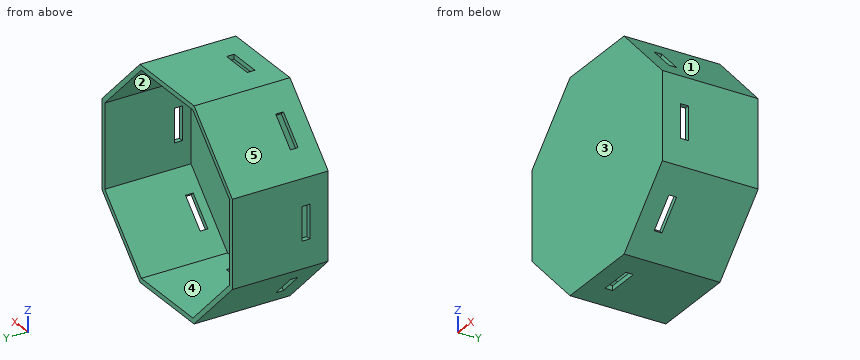
Autodesk Inventor part; units mm, degrees
ref_plane "YZ Plane" through (0, 0, 0) normal (1, 0, 0) x (0, 1, 0)
ref_plane "XZ Plane" through (0, 0, 0) normal (0, 1, 0) x (-1, 0, 0)
ref_plane "XY Plane" through (0, 0, 0) normal (0, 0, 1) x (1, 0, 0)
sketch "Skizze4" plane through (0, 0, 0) normal (0, 1, 0) x (-1, 0, 0)
  line L0 (77, 0) -> (-77, 0) construction
  line L1 (0, -77) -> (0, 77) construction
  line L2 (27, 37.5) -> (-27, 37.5) construction
  line L3 (-27, 37.5) -> (-27, -37.5) construction
  line L4 (-27, -37.5) -> (27, -37.5) construction
  line L5 (27, -37.5) -> (27, 37.5) construction
  line L6 (55, -22.7817) -> (22.7817, -55)
  line L7 (22.7817, -55) -> (-22.7817, -55)
  line L8 (-22.7817, -55) -> (-55, -22.7817)
  line L9 (-55, -22.7817) -> (-55, 22.7817)
  line L10 (-55, 22.7817) -> (-22.7817, 55)
  line L11 (-22.7817, 55) -> (22.7817, 55)
  line L12 (22.7817, 55) -> (55, 22.7817)
  line L13 (55, 22.7817) -> (55, -22.7817)
  line L14 (52.5, -21.7462) -> (21.7462, -52.5)
  line L15 (21.7462, -52.5) -> (-21.7462, -52.5)
  line L16 (-21.7462, -52.5) -> (-52.5, -21.7462)
  line L17 (-52.5, -21.7462) -> (-52.5, 21.7462)
  line L18 (-52.5, 21.7462) -> (-21.7462, 52.5)
  line L19 (-21.7462, 52.5) -> (21.7462, 52.5)
  line L20 (21.7462, 52.5) -> (52.5, 21.7462)
  line L21 (52.5, 21.7462) -> (52.5, -21.7462)
  point P0 (0, 0)
  point P1 (0, 0)
  dimension "d4" = 75
  dimension "d5" = 54
  dimension "d7" = 2.5
  dimension "d22" = 110
extrude "Extrusion2" add sketch "Skizze4" along normal blind 45
sketch "Skizze5" plane through (0, 0, 0) normal (0, -1, 0) x (1, 0, 0)
  line L0 (21.7462, -52.5) -> (-21.7462, -52.5)
  line L1 (-21.7462, -52.5) -> (-52.5, -21.7462)
  line L2 (-52.5, -21.7462) -> (-52.5, 21.7462)
  line L3 (-52.5, 21.7462) -> (-21.7462, 52.5)
  line L4 (-21.7462, 52.5) -> (21.7462, 52.5)
  line L5 (21.7462, 52.5) -> (52.5, 21.7462)
  line L6 (52.5, 21.7462) -> (52.5, -21.7462)
  line L7 (52.5, -21.7462) -> (21.7462, -52.5)
  line L8 (-55, -22.7817) -> (-22.7817, -55)
  line L9 (-22.7817, -55) -> (22.7817, -55)
  line L10 (22.7817, -55) -> (55, -22.7817)
  line L11 (55, -22.7817) -> (55, 22.7817)
  line L12 (55, 22.7817) -> (22.7817, 55)
  line L13 (22.7817, 55) -> (-22.7817, 55)
  line L14 (-22.7817, 55) -> (-55, 22.7817)
  line L15 (-55, 22.7817) -> (-55, -22.7817)
  point P0 (0, 0)
extrude "Extrusion3" add sketch "Skizze5" along normal blind 5 contours L0 L1 L2 L3 L4 L5 L6 L7 | L15 L14 L13 L12 L11 L10 L9 L8
sketch "Skizze7" plane through (55, 45, 22.7817) normal (1, 0, 0) x (0, 0, -1)
  line L0 (14.032, -36.43) -> (31.532, -36.43)
  line L1 (31.532, -36.43) -> (31.532, -40.43)
  line L2 (31.532, -40.43) -> (14.032, -40.43)
  line L3 (14.032, -40.43) -> (14.032, -36.43)
  line L4 (45.5635, -50) -> (0, -50)
  line L5 (45.5635, 0) -> (45.5635, -50)
  point P0 (22.7817, -45)
  dimension "d13" = 9.57
  dimension "d14" = 17.5
  dimension "d15" = 4
  dimension "d16" = 14.0315
extrude "Extrusion4" cut sketch "Skizze7" against normal through all
pattern_circular "Runde Anordnung1" count 8 over 360 about axis through (0, -10, 0) along (0, 1, 0) of "Extrusion4"
properties part number "Oktagon" material "Kst - PVC (rigid/white)"
Verification items for the finished model (mm, model axes). Face numbers are marked on the shaded views. A direction names the side the tool comes from. Coordinates: 2 decimals unless noted, no trailing zeros. Order: outer loops, then holes, each group sorted by start corner. A loop starts at its lowest first (then second) coordinate and runs counter-clockwise, first axis right, second up. Notation, with made-up numbers: (75, -5) -> (111, -5) arc R34 ccw to (111, 33) -> close; hole circle Ø1 at (-29.5, 17.5). An arc over 180 degrees is marked (long way). Use CSV: the item, a comma, the result in double quotes. Start each with the question number.
Q1. Depth check by flat-ended pin: P1, Ø5, axis at x = 36, y = 23.5, coming from the -Z side; P2, Ø12, axis at x = -9.5, z = 26, coming from the +Y side; P3, Ø2, axis at x = -54, y = 6.5, coming from the -Z side. Enter the tip coordinate at first touch or a pass-through.
Q2. Section check A-A, the plane z = 2. Record the cut outline in (x, y).
Q3. Section check B-B, the plane y = 36. Record the cut outline in (x, z), and give its area (3 significant figures).
Q4. Draft check along Z on the marked faces 3, 4 and 5. Enter one of: +Z half, -Z half, draft (parallel to the pull), parting line (faces both ways), or undercut.
Q5. Tool access check on the marked faces 1 and 2. Record the directions out of +Z, -Z, +X, -X, +Y, -Y that give a thin tool (end or side, any length) a straight path to the whole face; none if there is none.
Q6. Section check D-D, the plane z = 20. Record the cut outline in (x, y).
Q7. Section check C-C, the plane x = 40. Record the cut outline in (y, z), and give its area (3 significant figures).
Q8. Thickness scan on line 1 along Z through (x, y) = (13, 5); line 2 along Y through (x, z) = (-31.5, 40). Record the ranges inside material, lowest first.
Returned:
1,P1,"stops at z = -44.28"
1,P2,"stops at y = 0"
1,P3,"stops at z = -24.78"
2,outline,"(-55, -5) -> (55, -5) -> (55, 4.57) -> (52.5, 4.57) -> (52.5, 0) -> (-52.5, 0) -> (-52.5, 4.57) -> (-55, 4.57) -> close; (-55, 8.57) -> (-52.5, 8.57) -> (-52.5, 45) -> (-55, 45) -> close; (52.5, 8.57) -> (55, 8.57) -> (55, 45) -> (52.5, 45) -> close"
3,outline,"(-55, -22.78) -> (-22.78, -55) -> (22.78, -55) -> (55, -22.78) -> (55, 22.78) -> (22.78, 55) -> (-22.78, 55) -> (-55, 22.78) -> close; hole (-52.5, -21.75) -> (-21.75, -52.5) -> (21.75, -52.5) -> (52.5, -21.75) -> (52.5, 21.75) -> (21.75, 52.5) -> (-21.75, 52.5) -> (-52.5, 21.75) -> close"
3,area,"891 mm^2"
4,face 3,"draft"
4,face 4,"undercut"
4,face 5,"+Z half"
5,face 1,"+Z, +X, +Y, -Y"
5,face 2,"+Y"
6,outline,"(-55, -5) -> (55, -5) -> (55, 45) -> (52.5, 45) -> (52.5, 0) -> (-52.5, 0) -> (-52.5, 45) -> (-55, 45) -> close"
7,outline,"(-5, -37.78) -> (4.57, -37.78) -> (4.57, -34.25) -> (0, -34.25) -> (0, 34.25) -> (4.57, 34.25) -> (4.57, 37.78) -> (-5, 37.78) -> close; (8.57, -37.78) -> (45, -37.78) -> (45, -34.25) -> (8.57, -34.25) -> close; (8.57, 34.25) -> (45, 34.25) -> (45, 37.78) -> (8.57, 37.78) -> close"
7,area,"668 mm^2"
8,line 1,"z = -55 to -52.5, 52.5 to 55"
8,line 2,"y = -5 to 0"
